Build history of the part. All positions in model axes, mm. A direction names the side the tool comes from. Give positions to 0.01 mm unless a question says otherwise; leave off trailing zeros. Write each loop counter-clockwise with the first axis right and the second up, starting at its lowest first coordinate (ties: lowest second). Pieces come first, ordered by that corner, then holes. Notation, with made-up numbers: (64, 81.5) -> (108, 81.5) arc R12 cw to (108, 89.5) -> close; hole circle Ø4 at (31.5, 67.5). An arc over 180 degrees is marked (long way). Write item = value, one per line. Start each with the question number.
Q1. Saw through at C-C, the plane z = -6.25. List the corners of the cut face in (x, y), then the cut area to 3 significant figures.
Q2. Drop flat-ended pins along their axis: P1, Ø3.5, axis at x = 0, z = -7.5, coming from the -Y side; P2, Ø3.5, axis at y = 6.5, z = -7, coming from the +X side; P3, Ø0.8, axis at x = -8.5, y = 4.5, coming from the -Z side; P4, Ø0.8, axis at x = 11.5, z = -4.5, coming from the +Y side. Give the stop position or say it passes through.
Q3. Saw through at D-D, the plane y = 9.25. List the corners of the cut face in (x, z).
Q4. Saw through at A-A, the plane y = 1.5. List the corners of the cut face in (x, z).
Q5. Mould opens along X. For faces 5 (the face through (-13.3, 1.7, -4.2)), 6 (the face through (-5.306, 7.801, -8.665)), 7 (the face through (13.3, 1.7, -4.3)), 8 (the face through (-9, 0, -4)) say: pulls with the +X half, pulls with the -X half, needs draft (parallel to the pull), parting line crosses it, or undercut.
Q6. Wall check: line 1 (X direction, y = 9.25, z = -3); line 2 (Z direction, x = -8, y = 3.25); line 3 (Y direction, x = 2.75, z = -6). Give the ranges that are in metal, low to high.
Q7. Tool access for faces 1 (the face through (12, 3, -4)), 2 (the face through (-8, 2, -8.5)), 3 (the face through (-5, 9, -5.75)), 4 (the face through (7.5, 8, -7)): list every direction of +Z, -Z, +X, -X, +Y, -Y with a clear straight run to the whole face (end or side of a thin tool).
Q8. Saw through at B-B, the plane z = -4.25. List the corners of the cut face in (x, y).
Autodesk Inventor part; units mm, degrees
ref_plane "YZ Plane" through (0, 0, 0) normal (1, 0, 0) x (0, 1, 0)
ref_plane "XZ Plane" through (0, 0, 0) normal (0, 1, 0) x (-1, 0, 0)
ref_plane "XY Plane" through (0, 0, 0) normal (0, 0, 1) x (1, 0, 0)
sketch "Sketch1" plane through (0, 0, 0) normal (0, 1, 0) x (-1, 0, 0)
  line L0 (-7.55, 0) -> (0, 0)
  line L1 (0, -11.5) -> (-7.5, -11.5)
  line L2 (-7.5, 0) -> (-9.05, 0)
  line L3 (-9.05, -8.5) -> (0, -8.5)
  arc A0 (-9.05, 0) -> (-9.05, -8.5) centre (-9.05, -4.25) ccw
  line L4 (-7.55, 0) -> (-7.3, 0)
  line L5 (-7.3, -11.5) -> (-7.5, -11.5)
  line L6 (-7.55, 0) -> (-7.5, 0)
  line L7 (-7.5, -11.5) -> (-7.5, -11.5)
  line L8 (0, 0) -> (0, -11.5)
  line L9 (-7.5, 0) -> (-7.5, -8.5)
  line L10 (7.55, 0) -> (0, 0)
  line L11 (0, -11.5) -> (7.55, -11.5)
  line L12 (7.5, 0) -> (9.05, 0)
  line L13 (9.05, -8.5) -> (0, -8.5)
  arc A1 (9.05, -8.5) -> (9.05, 0) centre (9.05, -4.25) ccw
  line L14 (7.55, 0) -> (7.3, 0)
  line L15 (7.3, -11.5) -> (7.55, -11.5)
  line L16 (7.55, 0) -> (7.5, 0)
  line L17 (7.5, -11.5) -> (7.5, -11.5)
  line L18 (7.5, 0) -> (7.5, -11.5)
  line L19 (7.5, 0) -> (-7.5, 0)
  line L20 (-7.5, 0) -> (-7.5, -11.5)
  line L21 (-7.5, -11.5) -> (7.5, -11.5)
  line L22 (7.5, -11.5) -> (7.5, 0)
  line L23 (-7.5, -8.5) -> (-7.5, -11.5)
  point P0 (0, 0)
  point P1 (-7.55, -8.5)
  point P2 (-13.3, -4.25)
  point P3 (7.55, -8.5)
  point P4 (13.3, -4.25)
  point P5 (7.5, -8.5)
  dimension "d3" = 8.5
  dimension "d9" = 5.8
  dimension "d25" = 15
  dimension "d26" = 5.8
  dimension "d27" = 11.5
extrude "Extrusion1" add sketch "Sketch1" along normal blind 11.5 contours L0 L8 L3 L9 | L3 L8 L1 L20 | L10 L18 L13 L8 | L13 L18 L11 L8
sketch "Sketch2" plane through (-7.5, 0, 0) normal (0, 0, 1) x (1, 0, 0)
  line L0 (0, 0) -> (15, 0)
  line L1 (1, 0) -> (14, 0)
  line L2 (0, 11.5) -> (15, 11.5)
  line L3 (1.5, 0) -> (13.5, 0)
  line L4 (13.5, 0) -> (13.5, 10)
  line L5 (13.5, 10) -> (1.5, 10)
  line L6 (1.5, 10) -> (1.5, 0)
  point P0 (7.5, 0)
  point P1 (14, 10.5)
  point P2 (1, 10.5)
  dimension "d14" = 10.5
  dimension "d28" = 11.5
  dimension "d29" = 12
  dimension "d30" = 10
extrude "Extrusion3" add sketch "Sketch1" along normal blind 3 contours L0 L9 L3 A0 L2
extrude "Extrusion4" add sketch "Sketch1" along normal blind 3 contours L18 L10 L12 A1 L13
fillet "Fillet1" radius 3 1 edges at (-7.5, 3, -4.25)
fillet "Fillet2" radius 3 1 edges at (7.5, 3, -4.25)
extrude "Extrusion5" cut sketch "Sketch2" against normal blind 5.75
sketch "Sketch3" plane through (7.5, 0, -11.5) normal (0, 0, -1) x (-1, 0, 0)
  line L0 (1.5, 0) -> (13.5, 0)
  line L1 (13.5, 0) -> (13.5, 5)
  line L2 (10.8166, 10) -> (4.1834, 10)
  line L3 (1.5, 5) -> (1.5, 0)
  arc A0 (4.1834, 10) -> (1.5, 5) centre (7.5, 5) ccw
  arc A1 (13.5, 5) -> (10.8166, 10) centre (7.5, 5) ccw
  point P0 (7.5, 0)
  point P1 (13.5, 10)
  point P2 (1.5, 10)
  dimension "d33" = 12
  dimension "d34" = 10
extrude "Extrusion6" cut sketch "Sketch3" against normal blind 5.75
sketch "Sketch4" plane through (-7.5, 11.5, 0) normal (0, 0, 1) x (1, 0, 0)
  line L0 (1.5, -1.5) -> (13.5, -1.5)
  point P0 (7.5, -11.5)
  dimension "d40" = 10
properties part number "Motor_Bracket"
Report:
q1.outline = (-12.8, 0) -> (-6, 0) -> (-6, 5) arc R6 cw to (-3.32, 10) -> (3.32, 10) arc R6 cw to (6, 5) -> (6, 0) -> (12.8, 0) -> (12.8, 3) -> (10.5, 3) arc R3 cw to (7.5, 6) -> (7.5, 11.5) -> (-7.5, 11.5) -> (-7.5, 6) arc R3 cw to (-10.5, 3) -> (-12.8, 3) -> close
q1.area = 96.1 mm2
q2.P1 = 10
q2.P2 = 7.77
q2.P3 = through
q2.P4 = 3
q3.outline = (-7.5, -11.5) -> (-4.24, -11.5) -> (-4.24, -5.75) -> (-6, -5.75) -> (-6, 0) -> (-7.5, 0) -> close; (4.24, -11.5) -> (7.5, -11.5) -> (7.5, 0) -> (6, 0) -> (6, -5.75) -> (4.24, -5.75) -> close
q4.outline = (-9.05, -8.5) -> (-7.5, -8.5) -> (-7.5, -11.5) -> (-6, -11.5) -> (-6, 0) -> (-9.05, 0) arc R4.25 ccw to start; (6, -11.5) -> (7.5, -11.5) -> (7.5, -8.5) -> (9.05, -8.5) arc R4.25 ccw to (9.05, 0) -> (6, 0) -> close
q5.face_5 = pulls with the -X half
q5.face_6 = undercut
q5.face_7 = pulls with the +X half
q5.face_8 = needs draft
q6.line_1 = -7.5 to -6, 6 to 7.5
q6.line_2 = -8.5 to 0
q6.line_3 = 10 to 11.5
q7.face_1 = +Z, -Z, +X, +Y
q7.face_2 = -Z, -X, +Y, -Y
q7.face_3 = +Z, -Y
q7.face_4 = -Z, +X, +Y
q8.outline = (-13.3, 0) -> (-6, 0) -> (-6, 10) -> (6, 10) -> (6, 0) -> (13.3, 0) -> (13.3, 3) -> (10.5, 3) arc R3 cw to (7.5, 6) -> (7.5, 11.5) -> (-7.5, 11.5) -> (-7.5, 6) arc R3 cw to (-10.5, 3) -> (-13.3, 3) -> close
